Read the model definition and answer for the solid it produces. Units are mm, in the model's axes. Face numbers are marked on the shaded views. A direction names the side the tool comes from. Give positions to 0.01 mm unless a question says otherwise; leave off trailing zeros. Order: outer loops, then holes, each group sorted by start corner. A loop starts at its lowest first (then second) coordinate and runs counter-clockwise, first axis right, second up.
```python
from build123d import *

# Parameters (mm, degrees)
MAIN_BODY_EXTRUDE_DEPTH        = 19.05
HINGE_START                    = -26.043353817
HINGE_SHELL_OUTLINE_W          = 26.043353817
HINGE_SHELL_OUTLINE_H          = 33.02
HINGE_SHELL_DEPTH              = 52.086707634
GROOVE_START                   = -16.51
GROOVE_1_DEPTH                 = 1.27
GROOVE_START_2                 = 17.78
GROOVE_2_DEPTH                 = 1.27
SKETCH5_W                      = 19.05
SKETCH5_H                      = 19.05
TIBIA_CONNECTION_EXTRUDE_DEPTH = 31.75
SKETCH6_R                      = 2.54
PINHOLE_CUT_DEPTH              = 25.4
FILLET1_R                      = 1.27
CHAMFER1_SIZE                  = 2.54
FILLET2_R                      = 0.889


# Read off the part's stored shape, not the designer's step: Hinge Shell
with BuildPart() as part:
    # Sketch1 → Main Body Extrude (new, symmetric)
    with BuildSketch(Plane.XY):
        with BuildLine():
            Line((18.423353817, 0), (-18.423353817, 0))
            ThreePointArc((-18.423353817, 0), (0, 18.423353817), (18.423353817, 0))
        make_face()
        with BuildLine():
            Line((18.423353817, 0), (21.598353817, 0))
            ThreePointArc((21.598353817, 0), (0, 21.598353817), (-21.598353817, 0))
            Line((-21.598353817, 0), (-18.423353817, 0))
            ThreePointArc((-18.423353817, 0), (0, 18.423353817), (18.423353817, 0))
        make_face()
        with BuildLine():
            Line((24.138353817, 0), (21.598353817, 0))
            ThreePointArc((21.598353817, 0), (0, 21.598353817), (-21.598353817, 0))
            Line((-21.598353817, 0), (-24.138353817, 0))
            ThreePointArc((-24.138353817, 0), (0, 24.138353817), (24.138353817, 0))
        make_face()
        with BuildLine():
            ThreePointArc((24.138353817, 0), (0, 24.138353817), (-24.138353817, 0))
            Line((-24.138353817, 0), (-24.773353817, 0))
            ThreePointArc((-24.773353817, 0), (0, 24.773353817), (24.773353817, 0))
            Line((24.773353817, 0), (24.138353817, 0))
        make_face()
        with BuildLine():
            Line((27.313353817, 0), (24.773353817, 0))
            ThreePointArc((24.773353817, 0), (0, 24.773353817), (-24.773353817, 0))
            Line((-24.773353817, 0), (-27.313353817, 0))
            ThreePointArc((-27.313353817, 0), (0, 27.313353817), (27.313353817, 0))
        make_face()
        with BuildLine():
            Line((-27.313353817, 27.313353817), (-27.313353817, 0))
            ThreePointArc((-27.313353817, 0), (-19.313457701, 19.313457701), (0, 27.313353817))
            Line((0, 27.313353817), (-27.313353817, 27.313353817))
        make_face()
        with BuildLine():
            Line((27.313353817, 27.313353817), (0, 27.313353817))
            ThreePointArc((0, 27.313353817), (19.313457701, 19.313457701), (27.313353817, 0))
            Line((27.313353817, 0), (27.313353817, 27.313353817))
        make_face()
    extrude(amount=MAIN_BODY_EXTRUDE_DEPTH, both=True)

    # Hinge Shell outline → Hinge Shell (cut)
    with BuildSketch(Plane.YZ.offset(HINGE_START)):
        with Locations((13.021676908, 0)):
            Rectangle(HINGE_SHELL_OUTLINE_W, HINGE_SHELL_OUTLINE_H)
    extrude(amount=HINGE_SHELL_DEPTH, mode=Mode.SUBTRACT)

    # Sketch1<13> → Groove 1 (cut)
    with BuildSketch(Plane.XY.offset(GROOVE_START)):
        with BuildLine():
            Line((18.423353817, 0), (21.598353817, 0))
            ThreePointArc((21.598353817, 0), (0, 21.598353817), (-21.598353817, 0))
            Line((-21.598353817, 0), (-18.423353817, 0))
            ThreePointArc((-18.423353817, 0), (0, 18.423353817), (18.423353817, 0))
        make_face()
    extrude(amount=-GROOVE_1_DEPTH, mode=Mode.SUBTRACT)

    # Sketch1<14> → Groove 2 (cut)
    with BuildSketch(Plane.XY.offset(GROOVE_START_2)):
        with BuildLine():
            Line((18.423353817, 0), (21.598353817, 0))
            ThreePointArc((21.598353817, 0), (0, 21.598353817), (-21.598353817, 0))
            Line((-21.598353817, 0), (-18.423353817, 0))
            ThreePointArc((-18.423353817, 0), (0, 18.423353817), (18.423353817, 0))
        make_face()
    extrude(amount=-GROOVE_2_DEPTH, mode=Mode.SUBTRACT)

    # Sketch5 → Tibia Connection Extrude (add)
    with BuildSketch(Plane(origin=(0, 27.313353817, 0), x_dir=(1, 0, 0), z_dir=(0, 1, 0))):
        Rectangle(SKETCH5_W, SKETCH5_H)
    extrude(amount=TIBIA_CONNECTION_EXTRUDE_DEPTH)

    # Sketch6 → Pinhole Cut (cut)
    with BuildSketch(Plane.XY.offset(9.525)):
        with Locations((0, 46.363353817)):
            Circle(SKETCH6_R)
    extrude(amount=-PINHOLE_CUT_DEPTH, mode=Mode.SUBTRACT)

    # Fillet1
    fillet1_edges = [part.edges().sort_by_distance(p)[0] for p in [
        (-27.313353817, 27.313353817, 0),
        (27.313353817, 27.313353817, 0),
        (27.313353817, 13.656676909, 19.05),
        (0, 27.313353817, 19.05),
        (-27.313353817, 13.656676909, 19.05),
        (-27.313353817, 13.656676909, -19.05),
        (0, 27.313353817, -19.05),
        (27.313353817, 13.656676909, -19.05),
    ]]
    fillet(fillet1_edges, radius=FILLET1_R)

    # Chamfer1
    chamfer1_edges = [part.edges().sort_by_distance(p)[0] for p in [
        (0, 27.313353817, 9.525),
        (-9.525, 43.188353817, 9.525),
        (9.525, 27.313353817, 0),
        (9.525, 43.188353817, 9.525),
        (0, 59.063353817, -9.525),
        (9.525, 43.188353817, -9.525),
        (-9.525, 59.063353817, 0),
        (-9.525, 43.188353817, -9.525),
        (0, 59.063353817, 9.525),
        (9.525, 59.063353817, 0),
        (-9.525, 27.313353817, 0),
        (0, 27.313353817, -9.525),
    ]]
    chamfer(chamfer1_edges, length=CHAMFER1_SIZE)

    # Fillet2
    fillet2_edges = [part.edges().sort_by_distance(p)[0] for p in [
        (26.941379429, 0, -18.678025612),
        (0, 0, -19.05),
        (27.313353817, 0, 0),
        (0, 0, 19.05),
        (-27.313353817, 0, 0),
        (26.941379429, 0, 18.678025612),
        (-26.941379429, 0, 18.678025612),
        (-26.941379429, 0, -18.678025612),
    ]]
    fillet(fillet2_edges, radius=FILLET2_R)


solid = part.part
```
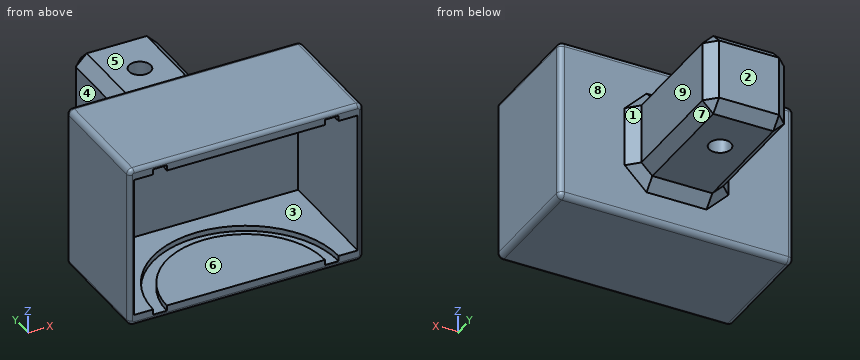
1) A tool of negligible diameter and unlimited length cuts with its end or side. For the marked faces 5, 6, 7, 8 and 9, from which of +Z, -Z, +X, -X, +Y, -Y can it reach the whole face along a straight path? Write none if from no direction.
Final values:
face 5: +Z, +X, -X, +Y
face 6: -Y
face 7: -Z, +X, +Y
face 8: +Y
face 9: +Z, -Z, +X, +Y
2) The part is cut by section D-D on x = 24. Determine the outline of the cut face in (y, z), and give its area (3 significant figures).
Final values:
outline: (0, -18.16) arc R0.89 ccw to (0.89, -19.05) - (26.04, -19.05) arc R1.27 ccw to (27.31, -17.78) - (27.31, 17.78) arc R1.27 ccw to (26.04, 19.05) - (0.89, 19.05) arc R0.89 ccw to (0, 18.16) - (0, 16.51) - (26.04, 16.51) - (26.04, -16.51) - (0, -16.51) - close
area: 180 mm2
3) The part is cut by section B-B on y = 25. Determine the outline of the cut face in (x, z), and give its area (3 significant figures).
Final values:
outline: (-27.31, -17.78) arc R1.27 ccw to (-26.04, -19.05) - (26.04, -19.05) arc R1.27 ccw to (27.31, -17.78) - (27.31, 17.78) arc R1.27 ccw to (26.04, 19.05) - (-26.04, 19.05) arc R1.27 ccw to (-27.31, 17.78) - close; hole (-26.04, -16.51) - (26.04, -16.51) - (26.04, 16.51) - (-26.04, 16.51) - close
area: 360 mm2
4) Given pin 1 (10 mm diameter, centred on x = -10, z = 6, fed in from -Y); pin 2 (3 mm diameter, centred on y = 28.5, z = 1, fed in from +X); pin 3 (10.5 mm diameter, centred on x = 10, z = 1, fed in from +Y); pin 4 (1 mm diameter, centred on x = -13, z = -8, fed in from +Y), each flat-ended and moving along its own axis, determine where each tip first touches the part or whether it passes through.
Final values:
pin 1: stops at y = 26.04
pin 2: stops at x = 26.88
pin 3: stops at y = 59.06
pin 4: stops at y = 27.31
5) Consider L1, parallel to X at y = 17.5, z = -12.5; L2, parallel to Y at x = 0, z = -1; L3, parallel to Z at x = 24, y = 22. Determine where each line is inside the solid, lowest interval first.
Final values:
L1: x = -27.31 to -26.04, 26.04 to 27.31
L2: y = 26.04 to 43.82, 48.9 to 59.06
L3: z = -19.05 to -16.51, 16.51 to 19.05
6) The part is cut by section C-C on z = -3.5. Determine the outline of the cut face in (x, y) (3 decimals).
Final values:
outline: (-27.313, 0.889) arc R0.889 ccw to (-26.424, 0) - (-26.043, 0) - (-26.043, 26.043) - (26.043, 26.043) - (26.043, 0) - (26.424, 0) arc R0.889 ccw to (27.313, 0.889) - (27.313, 26.043) arc R1.27 ccw to (26.043, 27.313) - (12.065, 27.313) - (9.525, 29.853) - (9.525, 56.523) - (6.985, 59.063) - (-6.985, 59.063) - (-9.525, 56.523) - (-9.525, 29.853) - (-12.065, 27.313) - (-26.043, 27.313) arc R1.27 ccw to (-27.313, 26.043) - close; hole circle Ø5.08 at (0, 46.363)
7) For a pull along X with two mould halves and no side action, classify the marked faces 1, 2, 3 and 4 as released by +X, released by -X, zero draft, split by the parting line, or undercut.
Final values:
face 1: released by +X
face 2: zero draft
face 3: undercut
face 4: released by -X
